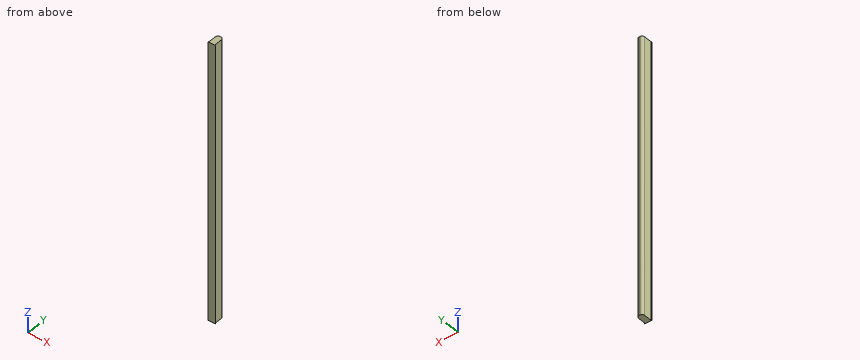
from build123d import *

# Parameters (mm, degrees)
RESSALTO_EXTRUS_O1_DEPTH = 115
FILETE1_R                = 1


with BuildPart() as part:
    # Esboço1 → Ressalto-extrusão1 (new body)
    with BuildSketch(Plane.XY):
        Polygon((-5.5, -1.198132677), (-5.5, -1.5), (-4.25, -1.5), (-4.25, 3), (-5.5, 3), align=None)
        with BuildLine():
            Line((-5.801867323, -1.5), (-5.5, -1.5))
            Line((-5.5, -1.5), (-5.5, -1.198132677))
            ThreePointArc((-5.5, -1.198132677), (-5.588414892, -1.411585108), (-5.801867323, -1.5))
        make_face()
        Polygon((-4.25, 3), (-4.25, -1.5), (-3, -1.5), (-3, -1.198132677), (-3, 3), align=None)
        with BuildLine():
            Line((-3, -1.198132677), (-3, -1.5))
            Line((-3, -1.5), (-2.698132677, -1.5))
            ThreePointArc((-2.698132677, -1.5), (-2.911585108, -1.411585108), (-3, -1.198132677))
        make_face()
    extrude(amount=RESSALTO_EXTRUS_O1_DEPTH)

    # Filete1
    filete1_edges = [part.edges().sort_by_distance(p)[0] for p in [
        (-3, 3, 57.5),
        (-5.5, 3, 57.5),
    ]]
    fillet(filete1_edges, radius=FILETE1_R)


solid = part.part
Here's how the part is built. I have some questions about the finished solid (model axes, mm). Coordinates: 2 decimals unless noted, no trailing zeros. Loops run counter-clockwise (first coordinate to the right, second up) from the corner with the lowest first, then second, coordinate; pieces in that order, holes last.
1. Imagine slicing it at A-A, the plane z = 16. Please give me the cut outline in (x, y).
2. I need wall thicknesses on L1, parallel to X at y = -0.7, z = 24; L2, parallel to Y at x = -3.95, z = 65; L3, parallel to Y at x = -3.5, z = 106. Which ranges of each line are inside material? Lowest first, please.
3. Imagine slicing it at B-B, the plane y = 0.9. Please give me the cut outline in (x, z), and give its area (4 significant figures).
4. For P1, Ø2.5, axis at y = 0.5, z = 46.5, coming from the -X side; P2, Ø1, axis at y = 2, z = 44.5, coming from the +X side, each with a flat end and sliding along its axis, tell me the tip position at first contact or that it passes through.
Taken from the geometry:
1. outline: (-5.8, -1.5) - (-2.7, -1.5) arc R0.3 cw to (-3, -1.2) - (-3, 2) arc R1 ccw to (-4, 3) - (-4.5, 3) arc R1 ccw to (-5.5, 2) - (-5.5, -1.2) arc R0.3 cw to start
2. L1: x = -5.5 to -3
2. L2: y = -1.5 to 3
2. L3: y = -1.5 to 2.87
3. outline: (-5.5, 0) - (-3, 0) - (-3, 115) - (-5.5, 115) - close
3. area: 287.5 mm2
4. P1: stops at x = -5.5
4. P2: stops at x = -3
